Design review of the part built by this model. Coordinates are the model's own, in mm. A direction names the side the tool comes from. Round coordinates to 2 decimals unless told otherwise and drop trailing zeros. Loops run counter-clockwise (first coordinate to the right, second up) from the corner with the lowest first, then second, coordinate; pieces in that order, holes last. Notation, with made-up numbers: (-19, -0.5) - (12, -0.5) arc R22 ccw to (12, 11.5) - close; hole circle Ø3 at (11.5, -27). An arc over 180 degrees is marked (long way). Return JSON: item names as keys, results as strings. Group by question number.
(1) Wall thickness on L1, parallel to Z at x = 0, y = 57; L2, parallel to X at y = 117, z = 43: over which ranges is each line inside the solid? List them lowest first. Write a range as [from, to].
(2) The part is to be moulded in two halves that separate along Y. For faces 1 (the cylindrical face through (-1.308, -7.139, 83.396)), 2 (the flat face through (3.978, -12.067, 74.591)), 3 (the cylindrical face through (-72.434, 81.619, -3.188)), say which applies: pulls with the +Y half, pulls with the -Y half, needs draft (parallel to the pull), parting line crosses it, or undercut.
(3) For faces 4 (the flat face through (-79.034, -28.766, 0.39)), 5 (the cylindrical face through (-83.396, 82.448, -3.67)), 6 (the flat face through (78.645, 28.624, 0.39)), list the 3-axis set-ups (+Z, -Z, +X, -X, +Y, -Y) from which the entire face can be reached by the end or side of a thin tool; tool diameter is ignored.
(4) We need section A-A, the plane y = 92. Write out the cut boundary in (x, z).
(5) Clearance check with flat-ended pins moving along their axes: pin 1 (2 mm diameter, centred on x = -45, y = 46.5, fed in from +Z); pin 2 (1 mm diameter, centred on y = 46, z = -27, fed in from -X); pin 3 (5 mm diameter, centred on y = 3, z = 19, fed in from -X); pin 4 (10 mm diameter, centred on x = 62.5, z = 1.5, fed in from -Y). State where each tip first meets the part, or that it passes through.
from build123d import *

# Parameters (mm, degrees)
SKETCH1_R                = 83.4771
SKETCH1_R_2              = 72.5043
BOSS_EXTRUDE1_DEPTH      = 152.4
BOSS_EXTRUDE1_DEPTH_BACK = 50.8
SKETCH4_W                = 203.2
SKETCH4_H                = 203.2
CUT_EXTRUDE1_DEPTH       = 152.4
SKETCH5_R                = 83.4771
SKETCH5_RX               = 77.157464469
SKETCH5_RY               = 72.5043
BOSS_EXTRUDE3_DEPTH      = 12.7


with BuildPart() as part:
    # Sketch1 → Boss-Extrude1 (new body, two sides)
    with BuildSketch(Plane(origin=(0, 0, 0), x_dir=(1, 0, 0), z_dir=(0, 1, 0))) as boss_extrude1_sk:
        Circle(SKETCH1_R)
        Circle(SKETCH1_R_2, mode=Mode.SUBTRACT)
    extrude(amount=BOSS_EXTRUDE1_DEPTH)
    extrude(boss_extrude1_sk.sketch, amount=-BOSS_EXTRUDE1_DEPTH_BACK)

    # Sketch4 → Cut-Extrude1 (cut)
    with BuildSketch(Plane(origin=(0, 0, 0), x_dir=(0, 0, -1), z_dir=(-0.342020143, 0.939692621, 0))):
        Rectangle(SKETCH4_W, SKETCH4_H)
    extrude(amount=-CUT_EXTRUDE1_DEPTH, mode=Mode.SUBTRACT)

    # Sketch5 → Boss-Extrude3 (add)
    with BuildSketch(Plane(origin=(0, 0, 0), x_dir=(0, 0, -1), z_dir=(-0.342020143, 0.939692621, 0))):
        Circle(SKETCH5_R)
        with Locations(Location((0, 0), (0, 0, -90))):
            Ellipse(SKETCH5_RX, SKETCH5_RY, mode=Mode.SUBTRACT)
    extrude(amount=-BOSS_EXTRUDE3_DEPTH)


solid = part.part
Solutions:
{
 "1": {"L1": "[-83.48, -72.5], [72.5, 83.48]", "L2": "[-71.55, -58.38], [58.38, 71.55]"},
 "2": {"face 1": "undercut", "face 2": "pulls with the -Y half", "face 3": "needs draft"},
 "3": {"face 4": "-Y", "face 5": "+Y", "face 6": "+X"},
 "4": {"outline": "circle Ø166.95 at (0, 0); hole circle Ø145.01 at (0, 0)"},
 "5": {"pin 1": "z = 70.94", "pin 2": "x = -79.16", "pin 3": "x = -81.83", "pin 4": "through"}
}
